The model under review builds one solid part; all positions refer to its coordinate system, in mm. A direction names the side the tool comes from. Coordinates: 2 decimals unless noted, no trailing zeros. Order: outer loops, then holes, each group sorted by start corner. A loop starts at its lowest first (then second) coordinate and runs counter-clockwise, first axis right, second up. Notation, with made-up numbers: (-4, 7.5) -> (4, 7.5) arc R22 cw to (4, 34.5) -> close; hole circle Ø11 at (45.5, 29). An arc over 180 degrees is marked (long way). Use one line per item in the form item = value.
from build123d import *

# Parameters (mm, degrees)
BOSS_EXTRUDE6_DEPTH   = 1778
BOSS_EXTRUDE6_2_DEPTH = 1778
BOSS_EXTRUDE6_3_DEPTH = 1778
BOSS_EXTRUDE6_4_DEPTH = 1778
SKETCH11_W            = 11.1125
SKETCH11_H            = 9.525
BOSS_EXTRUDE11_DEPTH  = 129.12986
SKETCH13_W            = 11.1125
SKETCH13_H            = 9.525
BOSS_EXTRUDE13_DEPTH  = 118.01736
SKETCH14_W            = 11.1125
SKETCH14_H            = 9.525
BOSS_EXTRUDE14_DEPTH  = 119.60486
SKETCH15_W            = 11.1125
SKETCH15_H            = 9.525
BOSS_EXTRUDE15_DEPTH  = 106.90486
LPATTERN1_COUNT       = 2
LPATTERN1_PITCH       = 381
LPATTERN2_COUNT       = 2
LPATTERN2_PITCH       = 635
LPATTERN3_COUNT       = 2
LPATTERN3_PITCH       = 1143
LPATTERN4_COUNT       = 2
LPATTERN4_PITCH       = 1768.475


with BuildPart() as part:
    # Sketch2 → Boss-Extrude6 (new body)
    with BuildSketch(Plane(origin=(0, 0, 0), x_dir=(1, 0, 0), z_dir=(0, 1, 0))):
        Polygon((0, 93.553663338), (-8.980256121, 84.573407217), (-7.857724106, 83.450875201), (0, 91.308599307), (7.857724106, 83.450875201), (8.980256121, 84.573407217), align=None)
    extrude(amount=BOSS_EXTRUDE6_DEPTH)



with BuildPart() as body_2:
    # Sketch2 → Boss-Extrude6 2 (new body)
    with BuildSketch(Plane(origin=(0, 0, 0), x_dir=(1, 0, 0), z_dir=(0, 1, 0))):
        Polygon((93.553663338, 0), (84.573407217, 8.980256121), (83.450875201, 7.857724106), (91.308599307, 0), (83.450875201, -7.857724106), (84.573407217, -8.980256121), align=None)
    extrude(amount=BOSS_EXTRUDE6_2_DEPTH)



with BuildPart() as body_3:
    # Sketch2 → Boss-Extrude6 3 (new body)
    with BuildSketch(Plane(origin=(0, 0, 0), x_dir=(1, 0, 0), z_dir=(0, 1, 0))):
        Polygon((0, -93.553663338), (8.980256121, -84.573407217), (7.857724106, -83.450875201), (0, -91.308599307), (-7.857724106, -83.450875201), (-8.980256121, -84.573407217), align=None)
    extrude(amount=BOSS_EXTRUDE6_3_DEPTH)



with BuildPart() as body_4:
    # Sketch2 → Boss-Extrude6 4 (new body)
    with BuildSketch(Plane(origin=(0, 0, 0), x_dir=(1, 0, 0), z_dir=(0, 1, 0))):
        Polygon((-93.553663338, 0), (-84.573407217, -8.980256121), (-83.450875201, -7.857724106), (-91.308599307, 0), (-83.450875201, 7.857724106), (-84.573407217, 8.980256121), align=None)
    extrude(amount=BOSS_EXTRUDE6_4_DEPTH)


with BuildPart() as body_3_1:
    add(body_3.part)

    add(body_4.part)  # Boss-Extrude11 merges body 4
    # Sketch11 → Boss-Extrude11 (add)
    with BuildSketch(Plane(origin=(-45.654299654, 0, -45.654299654), x_dir=(0.707106781, 0, -0.707106781), z_dir=(0.707106781, 0, 0.707106781))):
        with Locations((-59.008679751, 4.7625)):
            Rectangle(SKETCH11_W, SKETCH11_H)
    boss_extrude11 = extrude(amount=BOSS_EXTRUDE11_DEPTH)


with BuildPart() as body_2_1:
    add(body_2.part)

    add(body_3_1.part)  # Boss-Extrude13 merges body 3
    # Sketch13 → Boss-Extrude13 (add)
    with BuildSketch(Plane(origin=(-37.796575548, 0, 37.796575548), x_dir=(-0.707106781, 0, -0.707106781), z_dir=(0.707106781, 0, -0.707106781))):
        with Locations((-59.008679751, 4.7625)):
            Rectangle(SKETCH13_W, SKETCH13_H)
    boss_extrude13 = extrude(amount=BOSS_EXTRUDE13_DEPTH)


with BuildPart() as part_1:
    add(part.part)

    add(body_2_1.part)  # Boss-Extrude14 merges body 2
    # Sketch14 → Boss-Extrude14 (add)
    with BuildSketch(Plane(origin=(37.796575548, 0, 37.796575548), x_dir=(-0.707106781, 0, 0.707106781), z_dir=(-0.707106781, 0, -0.707106781))):
        with Locations((-59.008679751, 4.7625)):
            Rectangle(SKETCH14_W, SKETCH14_H)
    boss_extrude14 = extrude(amount=BOSS_EXTRUDE14_DEPTH)

    # Sketch15 → Boss-Extrude15 (add)
    with BuildSketch(Plane(origin=(37.796575548, 0, -37.796575548), x_dir=(0.707106781, 0, 0.707106781), z_dir=(-0.707106781, 0, 0.707106781))):
        with Locations((-59.008679751, 4.7625)):
            Rectangle(SKETCH15_W, SKETCH15_H)
    boss_extrude15 = extrude(amount=BOSS_EXTRUDE15_DEPTH)

    # LPattern1: Boss-Extrude11, Boss-Extrude13, Boss-Extrude14, Boss-Extrude15 ×2
    with Locations(*[(0, i * LPATTERN1_PITCH, 0) for i in range(1, LPATTERN1_COUNT)]):
        add(boss_extrude11)
        add(boss_extrude13)
        add(boss_extrude14)
        add(boss_extrude15)

    # LPattern2: Boss-Extrude11, Boss-Extrude13, Boss-Extrude14, Boss-Extrude15 ×2
    with Locations(*[(0, i * LPATTERN2_PITCH, 0) for i in range(1, LPATTERN2_COUNT)]):
        add(boss_extrude11)
        add(boss_extrude13)
        add(boss_extrude14)
        add(boss_extrude15)

    # LPattern3: Boss-Extrude11, Boss-Extrude13, Boss-Extrude14, Boss-Extrude15 ×2
    with Locations(*[(0, i * LPATTERN3_PITCH, 0) for i in range(1, LPATTERN3_COUNT)]):
        add(boss_extrude11)
        add(boss_extrude13)
        add(boss_extrude14)
        add(boss_extrude15)

    # LPattern4: Boss-Extrude11, Boss-Extrude13, Boss-Extrude14, Boss-Extrude15 ×2
    with Locations(*[(0, i * LPATTERN4_PITCH, 0) for i in range(1, LPATTERN4_COUNT)]):
        add(boss_extrude11)
        add(boss_extrude13)
        add(boss_extrude14)
        add(boss_extrude15)


solid = part_1.part
Item 1: Tool access review of faces 4 (the face through (38.326, 639.696, -37.267)), 5 (the face through (45.13, 4.7, 46.18)): name each direction out of +Z, -Z, +X, -X, +Y, -Y from which nothing blocks a thin tool from reaching the whole face with its end or side.
Results found:
face_4 = +Y, -Y
face_5 = +Z, +X, +Y, -Y
Item 2: We need section A-A (y = 945). Write out the cut boundary in (x, z).
Results found:
outline = (-93.55, 0) -> (-84.57, -8.98) -> (-83.45, -7.86) -> (-91.31, 0) -> (-83.45, 7.86) -> (-84.57, 8.98) -> close; (-8.98, -84.57) -> (0, -93.55) -> (8.98, -84.57) -> (7.86, -83.45) -> (0, -91.31) -> (-7.86, -83.45) -> close; (-8.98, 84.57) -> (-7.86, 83.45) -> (0, 91.31) -> (7.86, 83.45) -> (8.98, 84.57) -> (0, 93.55) -> close; (83.45, -7.86) -> (84.57, -8.98) -> (93.55, 0) -> (84.57, 8.98) -> (83.45, 7.86) -> (91.31, 0) -> close
Item 3: Draft analysis for pull direction Z (two halves, no side actions). For faces 1 (the face through (-42, 1778, 40)), 2 (the face through (-46.18, 1773.17, 45.13)), 3 (the face through (37.267, 4.696, 38.326)), state which applies: released by +Z, released by -Z, zero draft, split by the parting line, or undercut.
Results found:
face_1 = zero draft
face_2 = released by +Z
face_3 = undercut
Item 4: To check wall thickness, follow L1, parallel to Y at x = -60, z = -18 (3 decimals); L2, parallel to X at y = 1030, z = 1; L3, parallel to Z at x = 3, y = 1131.5. State the ranges of each line that lie inside material, in increasing order. Write a range as from..to.
Results found:
L1 = 0..9.525, 381..390.525, 635..644.525, 1143..1152.525, 1768.475..1778
L2 = -92.55..-90.31, 90.31..92.55
L3 = -90.55..-88.31, 88.31..90.55
Item 5: We need section B-B (z = 60). State how many separate pieces and enclosed holes the cut face has, plus the area to 3 significant figures.
Results found:
separate_pieces = 10
enclosed_holes = 0
area = 1,500 mm²
